Autodesk Inventor part; units mm, degrees
ref_plane "Work Plane1" through (0, 0, -15) normal (0, 0, 1) x (1, 0, 0)
ref_plane "YZ Plane" through (0, 0, 0) normal (1, 0, 0) x (0, 1, 0)
ref_plane "XZ Plane" through (0, 0, 0) normal (0, 1, 0) x (-1, 0, 0)
sketch "Sketch1" plane through (0, 0, 0) normal (0, 0, 1) x (1, 0, 0)
  line L0 (0, 0) -> (25, 0)
  line L1 (25, 0) -> (25, 40)
  line L2 (25, 40) -> (0, 40)
  line L3 (0, 40) -> (0, 0)
  dimension "d1" = 25
  dimension "d2" = 40
  dimension "d3" = 25
extrude "Extrusion1" add sketch "Sketch1" against normal blind 30
sketch "Sketch2" plane through (25, 0, 0) normal (1, 0, 0) x (0, 0, -1)
  line L0 (0, 0) -> (30, 0)
  circle A0 centre (15, 6.56) radius 2.46
extrude "Extrusion2" cut sketch "Sketch2" against normal blind 30
sketch "Sketch3" plane through (0, 0, 0) normal (-1, 0, 0) x (0, 0, 1)
  line L0 (0, 0) -> (-30, 0)
  line L1 (-25.05, 0) -> (-4.95, 0)
  line L2 (-4.95, 0) -> (-4.95, 33.12)
  line L3 (-4.95, 33.12) -> (-25.05, 33.12)
  line L4 (-25.05, 33.12) -> (-25.05, 0)
  dimension "d11" = 20.1
extrude "Extrusion3" cut sketch "Sketch3" against normal blind 20
sketch "Sketch4" plane through (0, 0, 0) normal (0, -1, 0) x (1, 0, 0)
  line L0 (20, -4.95) -> (20, -25.05)
  line L1 (20, -15) -> (25, -15)
  line L2 (25, 0) -> (25, -30)
  line L3 (20, -8.025) -> (25, -8.025)
  line L4 (25, -8.025) -> (25, -21.975)
  line L5 (25, -21.975) -> (20, -21.975)
  line L6 (20, -21.975) -> (20, -8.025)
  line L7 (20, -8.025) -> (25, -21.975) construction
  line L8 (25, -8.025) -> (20, -21.975) construction
  line L9 (25, -12.54) -> (25, -17.46)
  point P0 (0, 0)
  point P1 (22.5, -15)
  dimension "d14" = 13.95
extrude "Extrusion4" add sketch "Sketch4" along normal blind 15
sketch "Sketch5" plane through (20, 0, 0) normal (-1, 0, 0) x (0, 0, 1)
  circle A0 centre (-15, 6.56) radius 2.46
  circle A1 centre (-15, 6.56) radius 4.7025
  circle A2 centre (-15, 6.56) radius 2.46
  circle A3 centre (-15, 6.56) radius 2.46
  point P0 (0, 0)
  dimension "d17" = 9.405
extrude "Extrusion5" cut sketch "Sketch5" against normal blind 2.1
sketch "Sketch6" plane through (25, 0, 0) normal (1, 0, 0) x (0, 0, -1)
  circle A0 centre (15, 6.56) radius 4.7025
  line L0 (15, 6.56) -> (15, 23.56)
  circle A1 centre (15, 23.56) radius 2.46
  point P0 (0, 0)
  dimension "d20" = 17
  dimension "d21" = 4.92
extrude "Extrusion6" cut sketch "Sketch6" against normal blind 10 contours A1
sketch "Sketch7" plane through (20, 0, 0) normal (-1, 0, 0) x (0, 0, 1)
  circle A0 centre (-15, 23.56) radius 2.46
  circle A1 centre (-15, 23.56) radius 4.7025
  point P0 (0, 0)
  dimension "d24" = 9.405
extrude "Extrusion7" cut sketch "Sketch7" against normal blind 2.1
sketch "Sketch9" plane through (25, 0, 0) normal (1, 0, 0) x (0, 0, -1)
  circle A0 centre (15, 6.56) radius 2.46
  circle A1 centre (15, 6.56) radius 2.46
  circle A2 centre (15, 23.56) radius 2.46
  circle A3 centre (15, 23.56) radius 2.46
  line L0 (30, 40) -> (30, 0)
  line L1 (30, 0) -> (30, 40)
  line L2 (30, 40) -> (0, 40)
  line L3 (0, 40) -> (0, 0)
  line L4 (0, 0) -> (8.025, 0)
  line L5 (21.975, 0) -> (21.975, -15)
  line L6 (21.975, -15) -> (8.025, -15)
  line L7 (8.025, -15) -> (8.025, 0)
  line L8 (0, 0) -> (8.025, 0)
  line L9 (21.975, 0) -> (30, 0)
extrude "Extrusion8" add sketch "Sketch9" along normal blind 5
sketch "Sketch10" plane through (0, 40, 0) normal (0, 1, 0) x (1, 0, 0)
  line L0 (0, 30) -> (30, 30)
  line L1 (30, 0) -> (0, 0)
  line L2 (0, 30) -> (30, 30)
  line L3 (30, 30) -> (30, 0)
  line L4 (30, 0) -> (0, 0)
  line L5 (0, 0) -> (0, 30)
extrude "Extrusion9" add sketch "Sketch10" along normal blind 30
sketch "Sketch12" plane through (30, 0, 0) normal (1, 0, 0) x (0, 0, -1)
  circle A0 centre (15, 6.56) radius 2.46
  line L0 (15, 6.56) -> (15, 15.06)
  circle A1 centre (15, 15.06) radius 2.525
  point P0 (0, 0)
  dimension "d31" = 8.5
  dimension "d33" = 5.05
extrude "Extrusion10" cut sketch "Sketch12" against normal blind 30 contours A1
sketch "Sketch14" plane through (0, 0, 0) normal (0, 0, 1) x (1, 0, 0)
  line L0 (30, 70) -> (0, 70)
  line L1 (0, 70) -> (0, 85)
  line L2 (-15, 100) -> (-23, 100)
  line L3 (30, 0) -> (30, 70)
  line L4 (30, 109) -> (30, 70)
  arc A0 (0, 85) -> (-15, 100) centre (-15, 85) ccw
  line L5 (30, 105) -> (30, 100)
  line L6 (-23, 124) -> (15, 124)
  line L7 (-19, 122) -> (-23, 124)
  line L8 (-19, 122) -> (-15, 112)
  line L9 (-19, 102) -> (-23, 100)
  line L10 (-19, 102) -> (-15, 112)
  line L11 (30, 109) -> (15, 124)
  point P0 (0, 0)
  point P1 (0, 100)
  dimension "d47" = 30
  dimension "d54" = 15
extrude "Extrusion12" add sketch "Sketch14" against normal blind 30
sketch "Sketch15" plane through (0, 0, -25.05) normal (-1, 0, 0) x (0, 0, 1)
  line L0 (0, 33.12) -> (20.1, 33.12)
  line L1 (20.1, 33.12) -> (20.1, 0)
  line L2 (0, 33.12) -> (20.1, 33.12)
  line L3 (20.1, 33.12) -> (20.1, 31.1)
  line L4 (20.1, 31.1) -> (0, 31.1)
  line L5 (0, 31.1) -> (0, 33.12)
  point P0 (25.05, 0)
  dimension "d57" = 2.02
extrude "Extrusion13" add sketch "Sketch15" against normal blind 20
sketch "Sketch19" plane through (0, 0, 0) normal (0, 0, 1) x (1, 0, 0)
  arc A0 (0, 85) -> (-15, 100) centre (-15, 85) ccw
  arc A1 (0, 85) -> (-15, 100) centre (-15, 85) ccw
  line L0 (-15, 100) -> (-23, 100)
  line L1 (-15, 100) -> (-23, 100)
  line L2 (-23, 100) -> (-19, 102)
  line L3 (-23, 100) -> (-19, 102)
  line L4 (-19, 102) -> (-15, 112)
  line L5 (-19, 102) -> (-15, 112)
  line L6 (-15, 112) -> (-19, 122)
  line L7 (-15, 112) -> (-19, 122)
  line L8 (-19, 122) -> (-23, 124)
  line L9 (-19, 122) -> (-23, 124)
  line L10 (-23, 124) -> (15, 124)
  line L11 (-23, 124) -> (15, 124)
  line L12 (15, 124) -> (30, 109)
  line L13 (15, 124) -> (30, 109)
  line L14 (30, 109) -> (30, 85)
  line L15 (30, 0) -> (30, 109)
  line L16 (0, 85) -> (30, 85)
  point P0 (0, 0)
extrude "Extrusion14" add sketch "Sketch19" along normal blind 15
ref_plane "Work Plane1" through (0, 0, -15) normal (0, 0, 1) x (1, 0, 0)
mirror "Mirror1" about plane through (0, 0, -15) normal (0, 0, 1) of "Extrusion14"
properties part number "20mm_x_60mm"
Source: CAD feature listing. Evaluate the final solid. Frame: model axes, mm. A direction names the side the tool comes from. Coordinates: 2 decimals unless noted, no trailing zeros. Loops run counter-clockwise (first coordinate to the right, second up) from the corner with the lowest first, then second, coordinate; pieces in that order, holes last. Notation, with made-up numbers: (49.25, -3) -> (60.25, -3) arc R29 cw to (60.25, 21) -> close; hole circle Ø4 at (49, 5). An arc over 180 degrees is marked (long way). Answer in a Markdown table with one row per item. Add a question column.
Q1. Pull-direction query (Z, two-part tool) for faces 1 (the face through (30, 60, -15)), 2 (the face through (21.035, 27.525, -12.472)), 3 (the face through (25, -8, -8.025)); classes: pulls with the +Z half, pulls with the -Z half, needs draft (parallel to the pull), parting line crosses it, or undercut.
Q2. Reachability of faces 4 (the face through (20, 8, -20)), 5 (the face through (0, 53, -15)), 6 (the face through (15, 43, -30)), 7 (the face through (21.035, 7.973, -10.515)) from +Z, -Z, +X, -X, +Y, -Y: full face, straight path, thin tool, end or side. Return the list, or none.
Q3. Ray query, line 1 along Z through (x, y) = (13.5, 6); line 2 along Z through (x, y) = (24, 15); line 3 along Y through (x, z) = (26, -15) (3 decimals). Return the intervals inside material, ascending.
Q4. Section B-B on z = -15. Give the number of separate pieces and of enclosed holes in the cut face, and give its area (3 significant figures).
Q5. Contact query for flat-ended pins moving along their axis: pin 1 Ø1.5 at (y, z) = (30.5, -32) entering from +X; pin 2 Ø4 at (x, y) = (9, 60) entering from -Z; pin 3 Ø12 at (x, z) = (-14.5, -6) entering from -Y; pin 4 Ø3 at (y, z) = (25.5, -16) entering from -X. Output: stop coordinate, or through.
Q6. Section D-D on y = -4. Return the cut outline in (x, z) (3 decimals), and give its area (4 significant figures).
Q7. Section C-C on z = -35. Return the cut outline in (x, y), and give its area (3 significant figures).
Q8. Section A-A on y = 23.56. Return the cut outline in (x, z).
Computed values:
| question | item | result |
|---|---|---|
| 1 | face 1 | needs draft |
| 1 | face 2 | undercut |
| 1 | face 3 | pulls with the +Z half |
| 2 | face 4 | -X, -Y |
| 2 | face 5 | +Z, -Z, -X, -Y |
| 2 | face 6 | -Z, +X, -X, -Y |
| 2 | face 7 | -X |
| 3 | line 1 | z = -30 to -25.05, -4.95 to 0 |
| 3 | line 2 | z = -30 to -17.52, -12.48 to 0 |
| 3 | line 3 | y = -15 to 4.1, 9.02 to 12.535, 17.585 to 21.1, 26.02 to 113 |
| 4 | separate pieces | 4 |
| 4 | enclosed holes | 0 |
| 4 | area | 3,440 mm^2 |
| 5 | pin 1 | passes through |
| 5 | pin 2 | stops at z = -30 |
| 5 | pin 3 | stops at y = 98.52 |
| 5 | pin 4 | stops at x = 22.1 |
| 6 | outline | (20, -21.975) -> (30, -21.975) -> (30, -8.025) -> (20, -8.025) -> close |
| 6 | area | 139.5 mm^2 |
| 7 | outline | (-23, 100) -> (-15, 100) arc R15 cw to (0, 85) -> (30, 85) -> (30, 109) -> (15, 124) -> (-23, 124) -> (-19, 122) -> (-15, 112) -> (-19, 102) -> close |
| 7 | area | 1,530 mm^2 |
| 8 | outline | (0, -30) -> (30, -30) -> (30, -17.46) -> (22.1, -17.46) -> (22.1, -19.7) -> (20, -19.7) -> (20, -25.05) -> (0, -25.05) -> close; (0, -4.95) -> (20, -4.95) -> (20, -10.3) -> (22.1, -10.3) -> (22.1, -12.54) -> (30, -12.54) -> (30, 0) -> (0, 0) -> close |
